```python
from build123d import *

# Parameters (mm, degrees)
F1_DEPTH = 25
F2_R     = 1.6
F3_DEPTH = 25
F4_R     = 2


with BuildPart() as f1:
    # F0 (on Front) → F1 (new body)
    with BuildSketch(Plane.XZ):
        with BuildLine():
            ThreePointArc((-5.1, 0), (0, 5.1), (5.1, 0))
            Line((5.1, 0), (5.1, -13.9))
            Line((5.1, -13.9), (5.1, -18.9))
            Line((5.1, -18.9), (21.7700861394, -18.9))
            Line((21.7700861394, -18.9), (21.7700861394, -15.9))
            ThreePointArc((21.7700861394, -15.9), (21.1842997018, -14.4857864376), (19.7700861394, -13.9))
            Line((19.7700861394, -13.9), (12.1, -13.9))
            ThreePointArc((12.1, -13.9), (10.6857864376, -13.3142135624), (10.1, -11.9))
            Line((10.1, -11.9), (10.1, 0))
            ThreePointArc((10.1, 0), (0, 10.1), (-10.1, 0))
            Line((-10.1, 0), (-10.1, -11.9))
            ThreePointArc((-10.1, -11.9), (-10.6857864376, -13.3142135624), (-12.1, -13.9))
            Line((-12.1, -13.9), (-19.7700861394, -13.9))
            ThreePointArc((-19.7700861394, -13.9), (-21.1842997018, -14.4857864376), (-21.7700861394, -15.9))
            Line((-21.7700861394, -15.9), (-21.7700861394, -18.9))
            Line((-21.7700861394, -18.9), (-5.1, -18.9))
            Line((-5.1, -18.9), (-5.1, -13.9))
            Line((-5.1, -13.9), (-5.1, 0))
        make_face()
    extrude(amount=F1_DEPTH)

    # F2 (on face) → F3 (cut)
    with BuildSketch(Plane.XY.offset(-13.9)):
        with Locations((16.0536523908, -20.5)):
            Circle(F2_R)
        with Locations((16.0536523908, -4.5)):
            Circle(F2_R)
        with Locations((-16.0536523908, -4.5)):
            Circle(F2_R)
        with Locations((-16.0536523908, -20.5)):
            Circle(F2_R)
    extrude(amount=-F3_DEPTH, mode=Mode.SUBTRACT)

    # F4
    f4_edges = [f1.edges().sort_by_distance(p)[0] for p in [
        (-10.1, -25, -5.95),
        (-10.1, 0, -5.95),
    ]]
    fillet(f4_edges, radius=F4_R)


solid = f1.part
```
Geometry check sheet. Reference: the model listing, model coordinates, mm. A direction names the side the tool comes from. Coordinates: 2 decimals unless noted, no trailing zeros. Order: outer loops, then holes, each group sorted by start corner. A loop starts at its lowest first (then second) coordinate and runs counter-clockwise, first axis right, second up. Notation, with made-up numbers: M -3.75,-31 L 50.25,-31 A19 ccw 50.25,-16 Z; hole C 67,-36.75 d3. An arc over 180 degrees is marked long. Answer as a JSON object with one key per item and string values.
Q1. Cross-section at C-C on x = 0. Record the cut outline in (y, z).
Results are:
{"outline": "M -25,5.1 L 0,5.1 L 0,8.1 A2 ccw -2,10.1 L -23,10.1 A2 ccw -25,8.1 Z"}
Q2. Cross-section at B-B on y = -4.5. Record the cut outline in (x, z).
Results are:
{"outline": "M -21.77,-18.9 L -17.65,-18.9 L -17.65,-13.9 L -19.77,-13.9 A2 ccw -21.77,-15.9 Z; M -14.45,-18.9 L -5.1,-18.9 L -5.1,0 A5.1 cw 5.1,0 L 5.1,-18.9 L 14.45,-18.9 L 14.45,-13.9 L 12.1,-13.9 A2 cw 10.1,-11.9 L 10.1,0 A10.1 ccw -10.1,0 L -10.1,-11.9 A2 cw -12.1,-13.9 L -14.45,-13.9 Z; M 17.65,-18.9 L 21.77,-18.9 L 21.77,-15.9 A2 ccw 19.77,-13.9 L 17.65,-13.9 Z"}
Q3. Depth check by flat-ended pin: pin 1 Ø5 at (y, z) = (-2.5, -0.5) entering from +X; pin 2 Ø3 at (x, z) = (2.5, -7) entering from +Y; pin 3 Ø6 at (y, z) = (-17, -5) entering from -X; pin 4 Ø2 at (x, y) = (-5.5, -20.5) entering from +Z. Enter the tip coordinate at first touch or a pass-through.
Results are:
{"pin 1": "stops at x = 10.1", "pin 2": "passes through", "pin 3": "stops at x = -10.1", "pin 4": "stops at z = 9.04"}
Q4. Tool access check on faces 1 (the flat face through (5.1, -12, -9)), 2 (the cylindrical face through (-9.5, -0.57, -6.03)), 3 (the flat face through (16, -12, -13.9)), 4 (the cylindrical face through (15.88, -24.43, -14.5)), 5 (the cylindrical face through (15.88, -0.57, -14.5)). Record the directions out of +Z, -Z, +X, -X, +Y, -Y that give a thin tool (end or side, any length) a straight path to the whole face; none if there is none.
Results are:
{"face 1": "-Z, +Y, -Y", "face 2": "+Z, -X, +Y", "face 3": "+Z, +X, +Y, -Y", "face 4": "+Z, +X, -Y", "face 5": "+Z, +X, +Y"}
Q5. Cross-section at A-A on z = -4.5. Record the cut outline in (x, y), and give its area (3 significant figures).
Results are:
{"outline": "M -10.1,-23 A2 ccw -8.1,-25 L -5.1,-25 L -5.1,0 L -8.1,0 A2 ccw -10.1,-2 Z; M 5.1,-25 L 8.1,-25 A2 ccw 10.1,-23 L 10.1,-2 A2 ccw 8.1,0 L 5.1,0 Z", "area": "247 mm²"}
Q6. Scan lines: line 1 (X direction, y = -13.75, z = -17); line 2 (X direction, y = -19, z = -5); line 3 (X direction, y = -19.25, z = -17). Record each from-to range of solid material in increasing order.
Results are:
{"line 1": "x = -21.77 to -5.1, 5.1 to 21.77", "line 2": "x = -10.1 to -5.1, 5.1 to 10.1", "line 3": "x = -21.77 to -17.05, -15.05 to -5.1, 5.1 to 15.05, 17.05 to 21.77"}
Q7. Cross-section at D-D on y = -8.5. Record the cut outline in (x, z).
Results are:
{"outline": "M -21.77,-18.9 L -5.1,-18.9 L -5.1,0 A5.1 cw 5.1,0 L 5.1,-18.9 L 21.77,-18.9 L 21.77,-15.9 A2 ccw 19.77,-13.9 L 12.1,-13.9 A2 cw 10.1,-11.9 L 10.1,0 A10.1 ccw -10.1,0 L -10.1,-11.9 A2 cw -12.1,-13.9 L -19.77,-13.9 A2 ccw -21.77,-15.9 Z"}
